Geometry check sheet. Reference: the model listing, model coordinates, mm. Face numbers are marked on the shaded views. A direction names the side the tool comes from. Give positions to 0.01 mm unless a question says otherwise; leave off trailing zeros. Loops run counter-clockwise (first coordinate to the right, second up) from the corner with the lowest first, then second, coordinate; pieces in that order, holes last.
1. Release check for a two-part mould opening along Z. For the marked faces 3, 4, 5 and 6 record: +Z half, -Z half, draft (parallel to the pull), parting line (faces both ways), or undercut.
2. Go/stop test with a flat-tipped pin: pin 1 Ø5 at (x, z) = (-10, -19.5) entering from +Y. Record where the tip stops, or that it passes through.
3. Cross-section at A-A, the plane y = 2.25. Record the cut outline in (x, z).
4. Cross-section at C-C, the plane z = 23.5. Record the cut outline in (x, y).
5. Tool access check on the marked faces 1 and 2. Record the directions out of +Z, -Z, +X, -X, +Y, -Y that give a thin tool (end or side, any length) a straight path to the whole face; none if there is none.
6. Cross-section at B-B, the plane x = -2.5. Record the cut outline in (y, z), plus the area to 3 significant figures.
7. Material ranges on L1, parallel to X at y = 3, z = -20; L2, parallel to Z at x = -1, y = 2.25; L3, parallel to Y at x = -9, z = 18.5, recorded low to high.
from build123d import *

# Parameters (mm, degrees)
SKETCH_1_W      = 31
SKETCH_1_H      = 64
SKETCH_1_W_2    = 28.5
SKETCH_1_H_2    = 50
EXTRUDE_1_DEPTH = 15
SKETCH_2_W      = 31
SKETCH_2_H      = 64
EXTRUDE_2_DEPTH = 1
FILLET_1_R      = 3


with BuildPart() as part:
    # 草图1 → 凸台-拉伸1 (new body)
    with BuildSketch(Plane(origin=(0, 0, 0), x_dir=(1, 0, 0), z_dir=(0, 1, 0))):
        Rectangle(SKETCH_1_W, SKETCH_1_H)
        Rectangle(SKETCH_1_W_2, SKETCH_1_H_2, mode=Mode.SUBTRACT)
    extrude(amount=EXTRUDE_1_DEPTH)

    # 草图2 → 凸台-拉伸2 (add)
    with BuildSketch(Plane(origin=(0, 0, 0), x_dir=(1, 0, 0), z_dir=(0, 1, 0))):
        Rectangle(SKETCH_2_W, SKETCH_2_H)
    extrude(amount=-EXTRUDE_2_DEPTH)

    # 圆角1
    fillet_1_edges = [part.edges().sort_by_distance(p)[0] for p in [
        (15.5, 7, 32),
        (-15.5, 7, 32),
        (-15.5, 7, -32),
        (15.5, 7, -32),
    ]]
    fillet(fillet_1_edges, radius=FILLET_1_R)


solid = part.part
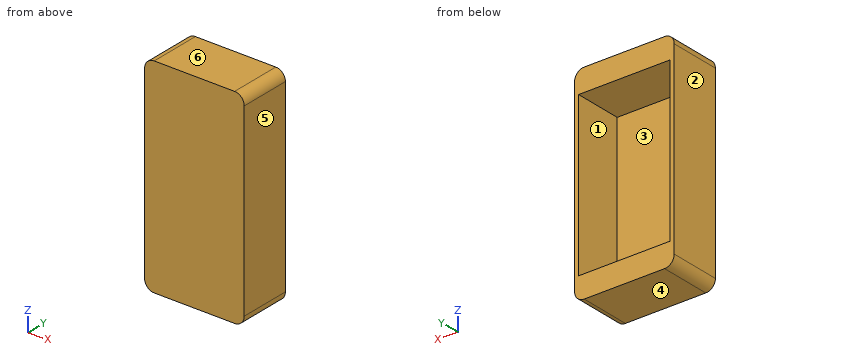
Result:
1. face 3: undercut
1. face 4: -Z half
1. face 5: draft
1. face 6: +Z half
2. pin 1: stops at y = 0
3. outline: (-15.5, -29) arc R3 ccw to (-12.5, -32) - (12.5, -32) arc R3 ccw to (15.5, -29) - (15.5, 29) arc R3 ccw to (12.5, 32) - (-12.5, 32) arc R3 ccw to (-15.5, 29) - close; hole (-14.25, -25) - (14.25, -25) - (14.25, 25) - (-14.25, 25) - close
4. outline: (-15.5, -1) - (15.5, -1) - (15.5, 15) - (14.25, 15) - (14.25, 0) - (-14.25, 0) - (-14.25, 15) - (-15.5, 15) - close
5. face 1: +Y
5. face 2: +Z, -Z, -X, +Y, -Y
6. outline: (-1, -32) - (15, -32) - (15, -25) - (0, -25) - (0, 25) - (15, 25) - (15, 32) - (-1, 32) - close
6. area: 274 mm2
7. L1: x = -15.5 to -14.25, 14.25 to 15.5
7. L2: z = -32 to -25, 25 to 32
7. L3: y = -1 to 0
